Design review of the part built by this model. Coordinates are the model's own, in mm. A direction names the side the tool comes from. Round coordinates to 2 decimals unless told otherwise and drop trailing zeros. Order: outer loops, then holes, each group sorted by start corner. A loop starts at its lowest first (then second) coordinate and runs counter-clockwise, first axis right, second up. Notation, with made-up numbers: M 7.5,-16 L 52.5,-16 A17 cw 52.5,9 Z; hole C 51.5,41 d4. An arc over 180 degrees is marked long. Use a Markdown table: item, result. Add a question column.
(1) Take a section at A-A (y = -30). Write out the cut boundary in (x, z).
(2) The part is to be moulded in two halves that separate along Y. For faces 1 (the face through (3, -1, -30)), 2 (the face through (4.5, 72.6, -2.5)), 3 (the face through (5, -90, 0)), say which applies: released by +Y, released by -Y, zero draft, split by the parting line, or undercut.
(3) For pin 1 (4.5 mm diameter, centred on y = -30, z = 25, fed in from +X); pin 2 (3.5 mm diameter, centred on y = 79, z = -1.5, fed in from +X); pin 3 (2 mm diameter, centred on x = 3.5, z = -25, fed in from -Y); pin 4 (2 mm diameter, centred on x = 4, z = 0, fed in from +Y), all flat-tipped, find the tip position at first contact; note any pin that passes through.
(4) Machinability: for faces 4 (the face through (4.26, -30.65, -26.57)), 5 (the face through (2, 74, 4)), which of the approach directions +Z, -Z, +X, -X, +Y, -Y give a long, thin tool a straight path to every point of the face, cutting with its end or side? Answer none if there is none.
(5) To check wall thickness, follow probe 1 along Z at (x, y) = (3.7, -30); probe 2 along Y at (x, z) = (5.25, -25); probe 3 along Z at (x, y) = (4.5, -80). State the ranges of each line that lie inside material, in increasing order. Write a range as from..to.
```python
from build123d import *

# Parameters (mm, degrees)
SKETCH_1_W                   = 60
SKETCH_1_H                   = 180
EXTRUDE_1_DEPTH              = 7
SKETCH_2_R                   = 5.5
CUT_EXTRUDE_1_DEPTH          = 5
SKETCH_3_R                   = 4.9
CUT_EXTRUDE_2_DEPTH          = 96
HOLE_WIZARD_M3_1_D           = 3.4
HOLE_WIZARD_M3_1_DEPTH       = 7.5
HOLE_WIZARD_M3_1_CSINK_D     = 6.3
HOLE_WIZARD_M3_1_CSINK_ANGLE = 90
HOLE_WIZARD_M3_1_TIP         = 1.021463052
F_1_0MM_3_REACH              = 184.617
F_1_0MM_3_BORE_R             = 1.35
F_1_0MM_2_D                  = 2.7
F_1_0MM_2_DEPTH              = 7.5
F_1_0MM_2_TIP                = 0.811161836
F_1_0MM_1_D                  = 2.7


with BuildPart() as part:
    # 草圖1 → 填料-伸長1 (new body)
    with BuildSketch(Plane(origin=(0, 0, 0), x_dir=(0, 0, -1), z_dir=(1, 0, 0))):
        Rectangle(SKETCH_1_W, SKETCH_1_H)
    extrude(amount=EXTRUDE_1_DEPTH)

    # 草圖2 → 除料-伸長1 (cut)
    with BuildSketch(Plane(origin=(7, 0, 0), x_dir=(0, 0, -1), z_dir=(1, 0, 0))):
        with Locations((0, 77.5)):
            Circle(SKETCH_2_R)
    extrude(amount=-CUT_EXTRUDE_1_DEPTH, mode=Mode.SUBTRACT)

    # 草圖3 → 除料-伸長2 (cut, through all)
    with BuildSketch(Plane(origin=(2, 0, 0), x_dir=(0, 0, -1), z_dir=(1, 0, 0))):
        with Locations((0, 77.5)):
            Circle(SKETCH_3_R)
    extrude(amount=-CUT_EXTRUDE_2_DEPTH, mode=Mode.SUBTRACT)

    # M3 錐坑平頭螺釘的錐孔1
    with Locations(Plane.ZY):
        with Locations((-25, -30), (0, -30), (25, -30)):
            CounterSinkHole(HOLE_WIZARD_M3_1_D / 2, HOLE_WIZARD_M3_1_CSINK_D / 2, depth=HOLE_WIZARD_M3_1_DEPTH, counter_sink_angle=HOLE_WIZARD_M3_1_CSINK_ANGLE)
            with Locations((0, 0, -(HOLE_WIZARD_M3_1_DEPTH + HOLE_WIZARD_M3_1_TIP / 2))):  # 118° drill point
                Cone(0, HOLE_WIZARD_M3_1_D / 2, HOLE_WIZARD_M3_1_TIP, mode=Mode.SUBTRACT)

    # Ø1.0mm 定位孔3 bore → Ø1.0mm 定位孔3 (cut, up to next)
    with BuildSketch(Plane(origin=(0, 90, 0), x_dir=(1, 0, 0), z_dir=(0, 1, 0)), mode=Mode.PRIVATE) as f_1_0mm_3_sk1:
        with Locations((4, 0)):
            Circle(F_1_0MM_3_BORE_R)
    f_1_0mm_3_tool1 = extrude(f_1_0mm_3_sk1.sketch, amount=-F_1_0MM_3_REACH, mode=Mode.PRIVATE) & part.part
    add(f_1_0mm_3_tool1.solids().sort_by_distance((4, 90, 0))[0], mode=Mode.SUBTRACT)

    # Ø1.0mm 定位孔2
    with Locations(Plane(origin=(0, -90, 0), x_dir=(-1, 0, 0), z_dir=(0, -1, 0))):
        with Locations((-3.5, 25), (-3.5, 0), (-3.5, -25)):
            Hole(F_1_0MM_2_D / 2, depth=F_1_0MM_2_DEPTH)
            with Locations((0, 0, -(F_1_0MM_2_DEPTH + F_1_0MM_2_TIP / 2))):  # 118° drill point
                Cone(0, F_1_0MM_2_D / 2, F_1_0MM_2_TIP, mode=Mode.SUBTRACT)

    # Ø1.0mm 定位孔1 (through all)
    with Locations(Plane.ZY):
        with Locations((25, -5), (25, -80), (-25, -80), (-25, -5)):
            Hole(F_1_0MM_1_D / 2)


solid = part.part
```
Verdict:
| question | item | result |
|---|---|---|
| 1 | outline | M 0,-30 L 7,-30 L 7,-26.7 L 1.45,-26.7 L 0,-28.15 Z; M 0,-21.85 L 1.45,-23.3 L 7,-23.3 L 7,-1.7 L 1.45,-1.7 L 0,-3.15 Z; M 0,3.15 L 1.45,1.7 L 7,1.7 L 7,23.3 L 1.45,23.3 L 0,21.85 Z; M 0,28.15 L 1.45,26.7 L 7,26.7 L 7,30 L 0,30 Z |
| 2 | face 1 | zero draft |
| 2 | face 2 | undercut |
| 2 | face 3 | released by -Y |
| 3 | pin 1 | stops at x = 7 |
| 3 | pin 2 | passes through |
| 3 | pin 3 | stops at y = -82.29 |
| 3 | pin 4 | stops at y = 72.09 |
| 4 | face 4 | +X, -X |
| 4 | face 5 | +X |
| 5 | probe 1 | z = -30..-26.7, -23.3..-1.7, 1.7..23.3, 26.7..30 |
| 5 | probe 2 | y = -90..-81.35, -78.65..-31.7, -28.3..-6.35, -3.65..90 |
| 5 | probe 3 | z = -30..-26.35, -23.65..23.65, 26.35..30 |
